The model under review builds one solid part; all positions refer to its coordinate system, in mm. Face numbers are marked on the shaded views. Coordinates: 2 decimals unless noted, no trailing zeros. Loops run counter-clockwise (first coordinate to the right, second up) from the corner with the lowest first, then second, coordinate; pieces in that order, holes last. Notation, with made-up numbers: M 14,19 L 57,19 A18 ccw 57,29 Z; hole C 19.5,-28 d11. An arc over 180 degrees is marked long. Use CSV: the item, a comma, the result in double quotes. Start each with the question number.
1. Add section D-D, the plane x = -8. Write out the cut boundary in (y, z).
2. For L1, parallel to Y at x = 7.5, z = 3; L2, parallel to X at y = -12.5, z = 2.3; L3, parallel to X at y = -12, z = 1.15, list the stretches that pass through material, from the lowest coordinate up.
3. Add section B-B, the plane z = 2.1. Write out the cut boundary in (x, y), then the cut area to 3 significant figures.
4. Add section A-A, the plane x = 0. Write out the cut boundary in (y, z).
5. Clearance check with flat-ended pins moving along their axes: P1, Ø4.5, axis at x = -7.5, y = -10.5, coming from the +Z side; P2, Ø1, axis at x = 4.5, z = 1, coming from the +Y side. State where each tip first meets the part, or that it passes through.
6. Draft analysis for pull direction Y (two halves, no side actions). For the marked faces 1, 2, 3 and 4, state which applies: +Y half, -Y half, draft (parallel to the pull), parting line (faces both ways), or undercut.
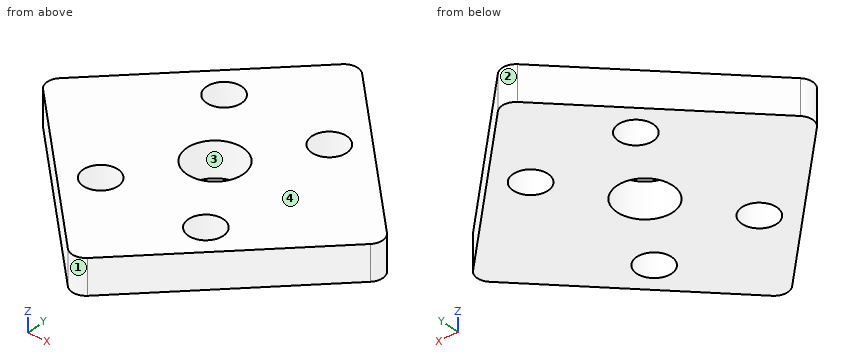
from build123d import *

# Parameters (mm, degrees)
EXTRUDE_1_DEPTH     = 5
SKETCH_2_R          = 4
CUT_EXTRUDE_1_DEPTH = 5
SKETCH_5_R          = 2.5
CUT_EXTRUDE_2_DEPTH = 36.355339059
FILLET_1_R          = 2


with BuildPart() as part:
    # 草图1 → 凸台-拉伸1 (new body)
    with BuildSketch(Plane.XY):
        Polygon((0, -24.748737342), (24.748737342, 0), (0, 24.748737342), (-24.748737342, 0), align=None)
    extrude(amount=EXTRUDE_1_DEPTH)

    # 草图2 → 切除-拉伸1 (cut)
    with BuildSketch(Plane.XY.offset(5)):
        Circle(SKETCH_2_R)
    extrude(amount=-CUT_EXTRUDE_1_DEPTH, mode=Mode.SUBTRACT)

    # 草图5 → 切除-拉伸2 (cut, through all)
    with BuildSketch(Plane.XY.offset(5)):
        with Locations((-7.5, 10.5)):
            Circle(SKETCH_5_R)
        with Locations(Location((7.5, 10.5, 0), (0, 0, 180))):
            Circle(SKETCH_5_R)
        with Locations((7.5, -10.5)):
            Circle(SKETCH_5_R)
        with Locations(Location((-7.5, -10.5, 0), (0, 0, 180))):
            Circle(SKETCH_5_R)
    extrude(amount=-CUT_EXTRUDE_2_DEPTH, mode=Mode.SUBTRACT)

    # 圆角1
    fillet_1_edges = [part.edges().sort_by_distance(p)[0] for p in [
        (-24.748737342, 0, 2.5),
        (0, 24.748737342, 2.5),
        (24.748737342, 0, 2.5),
        (0, -24.748737342, 2.5),
    ]]
    fillet(fillet_1_edges, radius=FILLET_1_R)


solid = part.part
Computed:
1,outline,"M -16.75,0 L -12.95,0 L -12.95,5 L -16.75,5 Z; M -8.05,0 L 8.05,0 L 8.05,5 L -8.05,5 Z; M 12.95,0 L 16.75,0 L 16.75,5 L 12.95,5 Z"
2,L1,"y = -17.25 to -13, -8 to 8, 13 to 17.25"
2,L2,"x = -12.25 to -9, -6 to 6, 9 to 12.25"
2,L3,"x = -12.75 to -9.5, -5.5 to 5.5, 9.5 to 12.75"
3,outline,"M -23.33,-1.41 L -1.41,-23.33 A2 ccw 1.41,-23.33 L 23.33,-1.41 A2 ccw 23.33,1.41 L 1.41,23.33 A2 ccw -1.41,23.33 L -23.33,1.41 A2 ccw Z; hole C -7.5,-10.5 d5; hole C -7.5,10.5 d5; hole C 0,0 d8; hole C 7.5,-10.5 d5; hole C 7.5,10.5 d5"
3,area,"1,090 mm^2"
4,outline,"M -23.92,0 L -4,0 L -4,5 L -23.92,5 Z; M 4,0 L 23.92,0 L 23.92,5 L 4,5 Z"
5,P1,"passes through"
5,P2,"stops at y = 20.75"
6,face 1,"-Y half"
6,face 2,"+Y half"
6,face 3,"undercut"
6,face 4,"draft"
